The listing builds one solid part. Answer for the finished solid, in the listing's coordinates (mm). Give positions to 0.01 mm unless a question says otherwise; leave off trailing zeros. Write each loop counter-clockwise with the first axis right and the second up, starting at its lowest first coordinate (ties: lowest second). Pieces come first, ordered by that corner, then holes. Notation, with made-up numbers: (-8.75, 22.25) -> (40.25, 22.25) arc R21 ccw to (40.25, 51.25) -> close; hole circle Ø8 at (11, 11). An arc over 180 degrees is marked (long way). Write each question's results on one line, items separated by ' | '. Start each with the question number.
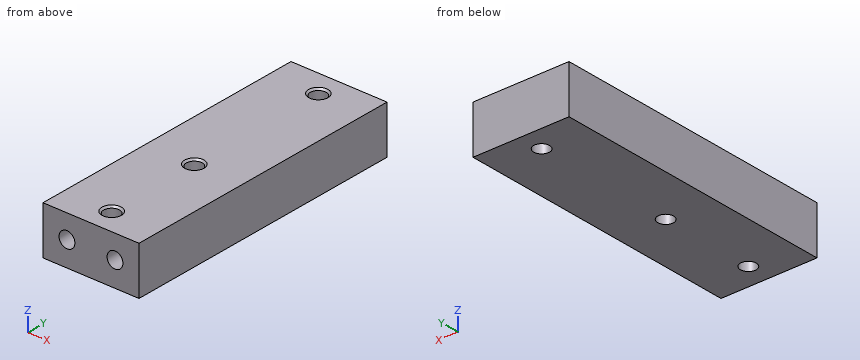
from build123d import *

# Parameters (mm, degrees)
SKIZZE1_W                          = 20
SKIZZE1_H                          = 60
AUFSATZ_LINEAR_AUSTRAGEN1_DEPTH    = 10
M4X0_7_GEWINDEBOHRUNG2_D           = 3.3
M4X0_7_GEWINDEBOHRUNG2_CSINK_D     = 4.05
M4X0_7_GEWINDEBOHRUNG2_CSINK_ANGLE = 90
M4_GEWINDEBOHRUNG1_D               = 3.3
M4_GEWINDEBOHRUNG1_DEPTH           = 30
M4_GEWINDEBOHRUNG1_TIP             = 0.991420021


with BuildPart() as part:
    # Skizze1 → Aufsatz-Linear austragen1 (new body)
    with BuildSketch(Plane.XY):
        with Locations((10, 30)):
            Rectangle(SKIZZE1_W, SKIZZE1_H)
    extrude(amount=AUFSATZ_LINEAR_AUSTRAGEN1_DEPTH)

    # M4x0.7 Gewindebohrung2 (through all)
    with Locations(Plane.XY.offset(10)):
        with Locations((10, 55), (10, 25), (10, 5)):
            CounterSinkHole(M4X0_7_GEWINDEBOHRUNG2_D / 2, M4X0_7_GEWINDEBOHRUNG2_CSINK_D / 2, counter_sink_angle=M4X0_7_GEWINDEBOHRUNG2_CSINK_ANGLE)

    # M4 Gewindebohrung1
    with Locations(Plane(origin=(0, 0, 0), x_dir=(-1, 0, 0), z_dir=(0, -1, 0))):
        with Locations((-15, -5.134624931), (-5, -5.134624931)):
            Hole(M4_GEWINDEBOHRUNG1_D / 2, depth=M4_GEWINDEBOHRUNG1_DEPTH)
            with Locations((0, 0, -(M4_GEWINDEBOHRUNG1_DEPTH + M4_GEWINDEBOHRUNG1_TIP / 2))):  # 118° drill point
                Cone(0, M4_GEWINDEBOHRUNG1_D / 2, M4_GEWINDEBOHRUNG1_TIP, mode=Mode.SUBTRACT)


solid = part.part
1. Section B-B (z = 1.5) is taken. Write down the section's boundary in (x, y), then the cut area to 3 significant figures.
2. Section A-A (x = 10) is taken. Write down the section's boundary in (y, z) (3 decimals), then the cut area to 3 significant figures.
3. Section C-C (y = 55) is taken. Write down the section's boundary in (x, z) (3 decimals), then the cut area to 3 significant figures.
4. Each of these flat-tipped pins is pushed along its axis until it touches: pin 1 Ø4 at (y, z) = (12.5, 6) entering from -X; pin 2 Ø2.5 at (x, z) = (15, 5.13) entering from -Y. Where does it stop, or does it pass through?
5. Consider probe 1 along X at (y, z) = (25, 5.25); probe 2 along X at (y, z) = (5, 7); probe 3 along Z at (x, y) = (5, 11.25). Determine where each line is inside the solid, lowest interval first. Write a range as [from, to].
6. Section D-D (y = 25) is taken. Write down the section's boundary in (x, z) (3 decimals), then the cut area to 3 significant figures.
Results:
1) outline: (0, 0) -> (20, 0) -> (20, 60) -> (0, 60) -> close; hole circle Ø3.3 at (10, 5); hole circle Ø3.3 at (10, 25); hole circle Ø3.3 at (10, 55) | area: 1,170 mm²
2) outline: (0, 0) -> (3.35, 0) -> (3.35, 9.625) -> (2.975, 10) -> (0, 10) -> close; (6.65, 0) -> (23.35, 0) -> (23.35, 9.625) -> (22.975, 10) -> (7.025, 10) -> (6.65, 9.625) -> close; (26.65, 0) -> (53.35, 0) -> (53.35, 9.625) -> (52.975, 10) -> (27.025, 10) -> (26.65, 9.625) -> close; (56.65, 0) -> (60, 0) -> (60, 10) -> (57.025, 10) -> (56.65, 9.625) -> close | area: 501 mm²
3) outline: (0, 0) -> (8.35, 0) -> (8.35, 9.625) -> (7.975, 10) -> (0, 10) -> close; (11.65, 0) -> (20, 0) -> (20, 10) -> (12.025, 10) -> (11.65, 9.625) -> close | area: 167 mm²
4) pin 1: stops at x = 0 | pin 2: stops at y = 30.24
5) probe 1: x = [0, 3.35], [6.65, 8.35], [11.65, 13.35], [16.65, 20] | probe 2: x = [0, 8.35], [11.65, 20] | probe 3: z = [0, 3.48], [6.78, 10]
6) outline: (0, 0) -> (8.35, 0) -> (8.35, 9.625) -> (7.975, 10) -> (0, 10) -> close; (11.65, 0) -> (20, 0) -> (20, 10) -> (12.025, 10) -> (11.65, 9.625) -> close; hole circle Ø3.3 at (5, 5.135); hole circle Ø3.3 at (15, 5.135) | area: 150 mm²
